Can you work these out from the model? Positions are in its coordinate system, mm. A direction names the side the tool comes from. Round coordinates to 2 decimals unless told otherwise and drop trailing zeros. Write each loop counter-clockwise with the first axis right and the second up, starting at its lowest first coordinate (ties: lowest second). Pieces come first, ordered by that corner, then holes. Notation, with made-up numbers: M 11.25,-33 L 66.25,-33 A25 cw 66.25,-2 Z; hole C -9.5,79.25 d11. An arc over 180 degrees is marked long. Answer in a Markdown table with one row per item. Add a question column.
(1) For faces 4 (the face through (-0.867, -3.905, 59.451)), 5 (the face through (-4, -2, 0)), 6 (the face through (3.233, -1.341, 3.301)), which set-ups out of +Z, -Z, +X, -X, +Y, -Y let a thin tool reach every point of the face, with its end or its side?
(2) Suppose I cut it at B-B, the plane z = 57. Write out the boundary of the cut face in (x, y), then the cut area to 3 significant figures.
(3) Suppose I cut it at A-A, the plane z = 27. Write out the boundary of the cut face in (x, y), then the cut area to 3 significant figures.
(4) If we mould it in two halves opening along X, with no side actions, what happens to faces 1 (the face through (0, 0, 63)), 2 (the face through (-1.19, -5.37, 25.64)), 3 (the face through (0.094, -0.424, 46.241))? For each: released by +X, released by -X, zero draft, split by the parting line, or undercut.
(5) I'm going to push flat-ended pins straight in: pin 1 (3 mm diameter, centred on x = 2, z = 23.5, fed in from +Y); pin 2 (3 mm diameter, centred on x = 3, z = 26, fed in from +Y); pin 3 (6.5 mm diameter, centred on x = 0, y = 0, fed in from -Z). Where does each tip first touch, or does it pass through?
(6) If I drill on probe 1 along Y at (x, z) = (-0.25, 33.5); probe 2 along Y at (x, z) = (0, 3.6); probe 3 along Z at (x, y) = (-1.25, -4.25), over which ranges is the centre line in solid material (lowest first)?
from build123d import *

# Parameters (mm, degrees)
SKETCH1_R                       = 5.5
BOSS_EXTRUDE1_DEPTH             = 52
SKETCH2_R                       = 4.5
BOSS_EXTRUDE2_DEPTH             = 4
SKETCH3_R                       = 4
BOSS_EXTRUDE3_DEPTH             = 7
F_5_0_5_DIAMETER_HOLE1_D        = 5
F_5_0_5_DIAMETER_HOLE1_DEPTH    = 45
F_5_0_5_DIAMETER_HOLE1_TIP      = 1.502151548
M8X1_0_TAPPED_HOLE1_D           = 7
M8X1_0_TAPPED_HOLE1_DEPTH       = 6
M8X1_0_TAPPED_HOLE1_CSINK_D     = 8.05
M8X1_0_TAPPED_HOLE1_CSINK_ANGLE = 90
M8X1_0_TAPPED_HOLE1_TIP         = 2.103012167


with BuildPart() as part:
    # Sketch1 → Boss-Extrude1 (new body)
    with BuildSketch(Plane.XY):
        Circle(SKETCH1_R)
    extrude(amount=BOSS_EXTRUDE1_DEPTH)

    # Sketch2 → Boss-Extrude2 (add)
    with BuildSketch(Plane.XY.offset(52)):
        Circle(SKETCH2_R)
    extrude(amount=BOSS_EXTRUDE2_DEPTH)

    # Sketch3 → Boss-Extrude3 (add)
    with BuildSketch(Plane.XY.offset(56)):
        Circle(SKETCH3_R)
    extrude(amount=BOSS_EXTRUDE3_DEPTH)

    # Ø5.0 (5) Diameter Hole1
    with Locations(Plane(origin=(0, 0, 0), x_dir=(-1, 0, 0), z_dir=(0, 0, -1))):
        with Locations((0, 0)):
            Hole(F_5_0_5_DIAMETER_HOLE1_D / 2, depth=F_5_0_5_DIAMETER_HOLE1_DEPTH)
            with Locations((0, 0, -(F_5_0_5_DIAMETER_HOLE1_DEPTH + F_5_0_5_DIAMETER_HOLE1_TIP / 2))):  # 118° drill point
                Cone(0, F_5_0_5_DIAMETER_HOLE1_D / 2, F_5_0_5_DIAMETER_HOLE1_TIP, mode=Mode.SUBTRACT)

    # M8x1.0 Tapped Hole1
    with Locations(Plane(origin=(0, 0, 0), x_dir=(-1, 0, 0), z_dir=(0, 0, -1))):
        with Locations((0, 0)):
            CounterSinkHole(M8X1_0_TAPPED_HOLE1_D / 2, M8X1_0_TAPPED_HOLE1_CSINK_D / 2, depth=M8X1_0_TAPPED_HOLE1_DEPTH, counter_sink_angle=M8X1_0_TAPPED_HOLE1_CSINK_ANGLE)
            with Locations((0, 0, -(M8X1_0_TAPPED_HOLE1_DEPTH + M8X1_0_TAPPED_HOLE1_TIP / 2))):  # 118° drill point
                Cone(0, M8X1_0_TAPPED_HOLE1_D / 2, M8X1_0_TAPPED_HOLE1_TIP, mode=Mode.SUBTRACT)


solid = part.part
Calculated:
| question | item | result |
|---|---|---|
| 1 | face 4 | +Z |
| 1 | face 5 | -Z, +X, -X, +Y, -Y |
| 1 | face 6 | -Z |
| 2 | outline | C 0,0 d8 |
| 2 | area | 50.3 mm² |
| 3 | outline | C 0,0 d11; hole C 0,0 d5 |
| 3 | area | 75.4 mm² |
| 4 | face 1 | zero draft |
| 4 | face 2 | split by the parting line |
| 4 | face 3 | undercut |
| 5 | pin 1 | y = 5.48 |
| 5 | pin 2 | y = 5.29 |
| 5 | pin 3 | z = 6.15 |
| 6 | probe 1 | -5.49 to -2.49, 2.49 to 5.49 |
| 6 | probe 2 | -5.5 to -3.5, 3.5 to 5.5 |
| 6 | probe 3 | 0 to 56 |
